Input: part model. Units: mm. Frame: model coordinates. A direction names the side the tool comes from. Give positions to 0.01 mm unless a question says otherwise; leave off trailing zeros. Write each loop counter-clockwise with the first axis right and the second up, starting at its lowest first coordinate (ties: lowest second). Pieces come first, ordered by that corner, then holes. Notation, with made-up numbers: (-31, 34) - (-3, 34) arc R16 ccw to (-3, 64) - close; hole circle Ø4 at (44.5, -13.75). An arc over 180 degrees is marked (long way). Answer as CSV lines item,"result". Start each with the question number.
from build123d import *

# Parameters (mm, degrees)
F4_DEPTH = 8.001


# Not quite as in the source:
# - a fillet or chamfer that OpenCascade refuses, or shapes differently, is made with other operations: its cross-section is extruded or revolved along the edge and cut away or added


with BuildPart() as f1:
    # F0 (on Front) → F1 (revolve)
    with BuildSketch(Plane.XZ):
        Polygon((-13, 0), (0, 0), (0, 8), (-13, 8), (-13, 7.5), (-8, 6.25), (-8, 1.75), (-13, 0.5), align=None)
    revolve(axis=Axis((0, 0, 4), (0, 0, 1)))

    # F2: fillet of radius 2 on 2 edges, made by hand

    # F2_s1 → F2_t2 (revolve, cut)
    with BuildSketch(Plane.XZ):
        with BuildLine():
            ThreePointArc((-13, 8), (-12.4961942947, 7.5030870148), (-11.8508805842, 7.212720146))
            Line((-11.8508805842, 7.212720146), (-13, 7.5))
            Line((-13, 7.5), (-13, 8))
        make_face()
    revolve(axis=Axis((0, 0, 7.5), (0, 0, 1)), mode=Mode.SUBTRACT)

    # F2_s3 → F2_t4 (revolve, cut)
    with BuildSketch(Plane.XZ):
        with BuildLine():
            ThreePointArc((-11.8508805842, 0.787279854), (-12.4961942947, 0.4969129852), (-13, 0))
            Line((-13, 0), (-13, 0.5))
            Line((-13, 0.5), (-11.8508805842, 0.787279854))
        make_face()
    revolve(axis=Axis((0, 0, 0.5), (0, 0, 1)), mode=Mode.SUBTRACT)

    # F3 (on Top) → F4 (cut, through all)
    with BuildSketch(Plane.XY):
        Polygon((6.808574619, 1.5439145703), (3.722676821, 5.9061017456), (-1.5439145703, 6.808574619), (-5.9061017456, 3.722676821), (-6.808574619, -1.5439145703), (-3.722676821, -5.9061017456), (1.5439145703, -6.808574619), (5.9061017456, -3.722676821), align=None)
    extrude(amount=F4_DEPTH, mode=Mode.SUBTRACT)


solid = f1.part
1) Contact query for flat-ended pins moving along their axis: P1, Ø1, axis at y = -4, z = 4, coming from the -X side; P2, Ø3, axis at x = -7.5, z = 6, coming from the -Y side. Output: stop coordinate, or through.
2) Cut plane A-A on z = 4. Output: boundary loops of the cut face in (x, y), and give its area (3 significant figures).
3) Reachability of faces 4 (the flat face through (-3.69, 5.29, 3.94)), 5 (the flat face through (3, -6, 0)), 6 (the cylindrical face through (1.73, 7.81, 3.97)) from +Z, -Z, +X, -X, +Y, -Y: full face, straight path, thin tool, end or side. Return the list, or none.
4) Cut plane B-B on y = 0. Output: boundary loops of the cut face in (x, z), and give its area (3 significant figures).
5) Pull-direction query (X, two-part tool) for faces 1 (the conical face through (-7.86, -2.48, 1.69)), 2 (the flat face through (-1.13, -6.35, 3.94)), 3 (the flat face through (-6, -3, 8)); classes: +X half, -X half, draft (parallel to the pull), parting line (faces both ways), or undercut.
6) Material intervals for line 1 (Y direction, x = -4.75, z = 5); line 2 (X direction, y = 4.5, z = 4.75); line 3 (X direction, y = 3, z = 2.5), sorted ascending. Write a range as from..to.
7) Cut plane D-D on z = 1.25. Output: boundary loops of the cut face in (x, y), and give its area (3 significant figures).
Numbers:
1,P1,"stops at x = -7.19"
1,P2,"stops at y = -10.18"
2,outline,"circle Ø16 at (0, 0); hole (-6.81, -1.54) - (-3.72, -5.91) - (1.54, -6.81) - (5.91, -3.72) - (6.81, 1.54) - (3.72, 5.91) - (-1.54, 6.81) - (-5.91, 3.72) - close"
2,area,"63.2 mm²"
3,face 4,"+Z, -Z"
3,face 5,"-Z, +X, -X, +Y, -Y"
3,face 6,"none"
4,outline,"(-13, 0) - (-6.54, 0) - (-6.54, 8) - (-13, 8) arc R2 ccw to (-11.85, 7.21) - (-8, 6.25) - (-8, 1.75) - (-11.85, 0.79) arc R2 ccw to start; (6.54, 0) - (13, 0) arc R2 ccw to (11.85, 0.79) - (8, 1.75) - (8, 6.25) - (11.85, 7.21) arc R2 ccw to (13, 8) - (6.54, 8) - close"
4,area,"45.1 mm²"
5,face 1,"parting line"
5,face 2,"undercut"
5,face 3,"draft"
6,line 1,"y = -6.44..-4.45, 4.54..6.44"
6,line 2,"x = -6.61..-4.81, 4.72..6.61"
6,line 3,"x = -7.42..-6.03, 5.78..7.42"
7,outline,"circle Ø20 at (0, 0); hole (-6.81, -1.54) - (-3.72, -5.91) - (1.54, -6.81) - (5.91, -3.72) - (6.81, 1.54) - (3.72, 5.91) - (-1.54, 6.81) - (-5.91, 3.72) - close"
7,area,"176 mm²"
